The model under review builds one solid part; all positions refer to its coordinate system, in mm. A direction names the side the tool comes from. Give positions to 0.01 mm unless a question says otherwise; leave off trailing zeros. Order: outer loops, then holes, each group sorted by start corner. A loop starts at its lowest first (then second) coordinate and runs counter-clockwise, first axis right, second up. Notation, with made-up numbers: (24.5, -2.75) -> (57.5, -2.75) arc R15 cw to (57.5, 9.25) -> close; hole circle Ø10 at (24, 55). An arc over 180 degrees is marked (long way). Use one line per item in the form item = value.
```python
from build123d import *

# Parameters (mm, degrees)
SKETCH1_W           = 35
SKETCH1_H           = 35
BOSS_EXTRUDE1_DEPTH = 9
SKETCH2_W           = 2
SKETCH2_H           = 35
SKETCH2_W_2         = 1.8
CUT_EXTRUDE1_DEPTH  = 3
SKETCH3_W           = 35
SKETCH3_H           = 3
CUT_EXTRUDE2_DEPTH  = 3
SKETCH4_W           = 7
SKETCH4_H           = 2.65
CUT_EXTRUDE3_DEPTH  = 51.309044912
SKETCH5_W           = 32
SKETCH5_H           = 3
CUT_EXTRUDE4_DEPTH  = 3
SKETCH6_W           = 17.8
SKETCH6_H           = 2
CUT_EXTRUDE5_DEPTH  = 3
SKETCH7_W           = 1.5
SKETCH7_H           = 2.079992284
SKETCH7_H_2         = 2.089639239
SKETCH7_H_3         = 2.130315237
SKETCH7_H_4         = 2.284421
SKETCH7_H_5         = 1.923722947
SKETCH7_H_6         = 2.10231694
SKETCH7_H_7         = 1.921766709
CUT_EXTRUDE6_DEPTH  = 3
SKETCH8_W           = 1.5
SKETCH8_H           = 1.855781426
SKETCH8_H_2         = 1.933933062
SKETCH8_H_3         = 1.973134408
SKETCH8_H_4         = 2.021952678
SKETCH8_H_5         = 2.006089453
SKETCH8_H_6         = 2.101240168
SKETCH8_H_7         = 2.045740356
CUT_EXTRUDE7_DEPTH  = 3
SKETCH9_W           = 32
SKETCH9_H           = 3
CUT_EXTRUDE9_DEPTH  = 3
SKETCH11_W          = 29
SKETCH11_H          = 3
CUT_EXTRUDE10_DEPTH = 3


with BuildPart() as part:
    # Sketch1 → Boss-Extrude1 (new body)
    with BuildSketch(Plane(origin=(0, 0, 0), x_dir=(1, 0, 0), z_dir=(0, 1, 0))):
        with Locations((17.5, 17.5)):
            Rectangle(SKETCH1_W, SKETCH1_H)
    extrude(amount=BOSS_EXTRUDE1_DEPTH)

    # Sketch2 → Cut-Extrude1 (cut)
    with BuildSketch(Plane(origin=(0, 9, 0), x_dir=(1, 0, 0), z_dir=(0, 1, 0))):
        with Locations((34, 17.5)):
            Rectangle(SKETCH2_W, SKETCH2_H)
        with Locations((30.6, 17.5)):
            Rectangle(SKETCH2_W_2, SKETCH2_H)
        with Locations((27.3, 17.5)):
            Rectangle(SKETCH2_W_2, SKETCH2_H)
        with Locations((1, 17.5)):
            Rectangle(SKETCH2_W, SKETCH2_H)
        with Locations((4.4, 17.5)):
            Rectangle(SKETCH2_W_2, SKETCH2_H)
        with Locations((7.7, 17.5)):
            Rectangle(SKETCH2_W_2, SKETCH2_H)
    extrude(amount=-CUT_EXTRUDE1_DEPTH, mode=Mode.SUBTRACT)

    # Sketch3 → Cut-Extrude2 (cut)
    with BuildSketch(Plane(origin=(35, 0, 0), x_dir=(0, 0, -1), z_dir=(1, 0, 0))):
        with Locations((17.5, 2)):
            Rectangle(SKETCH3_W, SKETCH3_H)
    extrude(amount=-CUT_EXTRUDE2_DEPTH, mode=Mode.SUBTRACT)

    # Sketch4 → Cut-Extrude3 (cut, through all)
    with BuildSketch(Plane.XY):
        with Locations((22.9, 7.387674937)):
            Rectangle(SKETCH4_W, SKETCH4_H)
        with Locations((12.1, 7.318212489)):
            Rectangle(SKETCH4_W, SKETCH4_H)
    extrude(amount=-CUT_EXTRUDE3_DEPTH, mode=Mode.SUBTRACT)

    # Sketch5 → Cut-Extrude4 (cut)
    with BuildSketch(Plane.XY):
        with Locations((16, 2)):
            Rectangle(SKETCH5_W, SKETCH5_H)
    extrude(amount=-CUT_EXTRUDE4_DEPTH, mode=Mode.SUBTRACT)

    # Sketch6 → Cut-Extrude5 (cut)
    with BuildSketch(Plane(origin=(0, 9, 0), x_dir=(1, 0, 0), z_dir=(0, 1, 0))):
        with Locations((17.5, 4)):
            Rectangle(SKETCH6_W, SKETCH6_H)
        with Locations((17.5, 9)):
            Rectangle(SKETCH6_W, SKETCH6_H)
        with Locations((17.5, 31)):
            Rectangle(SKETCH6_W, SKETCH6_H)
        with Locations((17.5, 26)):
            Rectangle(SKETCH6_W, SKETCH6_H)
    extrude(amount=-CUT_EXTRUDE5_DEPTH, mode=Mode.SUBTRACT)

    # Sketch7 → Cut-Extrude6 (cut)
    with BuildSketch(Plane(origin=(0, 9, 0), x_dir=(1, 0, 0), z_dir=(0, 1, 0))):
        with Locations((6.05, 25.936938184)):
            Rectangle(SKETCH7_W, SKETCH7_H)
        with Locations((2.75, 25.861771744)):
            Rectangle(SKETCH7_W, SKETCH7_H_2)
        with Locations((6.05, 30.892822657)):
            Rectangle(SKETCH7_W, SKETCH7_H_3)
        with Locations((2.75, 30.815769775)):
            Rectangle(SKETCH7_W, SKETCH7_H_4)
        with Locations((28.95, 30.996118802)):
            Rectangle(SKETCH7_W, SKETCH7_H_5)
        with Locations((32.25, 30.996118802)):
            Rectangle(SKETCH7_W, SKETCH7_H_5)
        with Locations((28.95, 25.828744005)):
            Rectangle(SKETCH7_W, SKETCH7_H_6)
        with Locations((32.25, 25.738468889)):
            Rectangle(SKETCH7_W, SKETCH7_H_7)
    extrude(amount=-CUT_EXTRUDE6_DEPTH, mode=Mode.SUBTRACT)

    # Sketch8 → Cut-Extrude7 (cut)
    with BuildSketch(Plane(origin=(0, 9, 0), x_dir=(1, 0, 0), z_dir=(0, 1, 0))):
        with Locations((28.95, 9.105526505)):
            Rectangle(SKETCH8_W, SKETCH8_H)
        with Locations((32.25, 9.105526505)):
            Rectangle(SKETCH8_W, SKETCH8_H)
        with Locations((32.25, 3.949699522)):
            Rectangle(SKETCH8_W, SKETCH8_H_2)
        with Locations((28.95, 3.95623308)):
            Rectangle(SKETCH8_W, SKETCH8_H_3)
        with Locations((6.05, 3.923953213)):
            Rectangle(SKETCH8_W, SKETCH8_H_4)
        with Locations((6.05, 9.030372491)):
            Rectangle(SKETCH8_W, SKETCH8_H_5)
        with Locations((2.75, 8.982797134)):
            Rectangle(SKETCH8_W, SKETCH8_H_6)
        with Locations((2.75, 3.769333302)):
            Rectangle(SKETCH8_W, SKETCH8_H_7)
    extrude(amount=-CUT_EXTRUDE7_DEPTH, mode=Mode.SUBTRACT)

    # Sketch9 → Cut-Extrude9 (cut)
    with BuildSketch(Plane(origin=(0, 0, -35), x_dir=(-1, 0, 0), z_dir=(0, 0, -1))):
        with Locations((-16, 2)):
            Rectangle(SKETCH9_W, SKETCH9_H)
    extrude(amount=-CUT_EXTRUDE9_DEPTH, mode=Mode.SUBTRACT)

    # Sketch11 → Cut-Extrude10 (cut)
    with BuildSketch(Plane.ZY):
        with Locations((-17.5, 2)):
            Rectangle(SKETCH11_W, SKETCH11_H)
    extrude(amount=-CUT_EXTRUDE10_DEPTH, mode=Mode.SUBTRACT)


solid = part.part
```
1. Add section A-A on x = 8. Give the boundary of the cut face in (y, z), then the cut area to 3 significant figures.
Values:
outline = (0, -35) -> (0.5, -35) -> (0.5, -32) -> (3.5, -32) -> (3.5, -35) -> (6, -35) -> (6, 0) -> (3.5, 0) -> (3.5, -3) -> (0.5, -3) -> (0.5, 0) -> (0, 0) -> close
area = 192 mm^2
2. Add section B-B on x = 15. Count the separate pieces of the cut face and the enclosed holes in it, then the cut area to 3 significant figures.
Values:
separate_pieces = 6
enclosed_holes = 0
area = 201 mm^2
3. Tool access review of faces 4 (the face through (32, 8, -26.699)), 5 (the face through (19.4, 7, -33)), 6 (the face through (3.5, 8, -28)): name each direction out of +Z, -Z, +X, -X, +Y, -Y from which nothing blocks a thin tool from reaching the whole face with its end or side.
Values:
face_4 = +X, -X, +Y
face_5 = +Z, -Z
face_6 = +Z, -Z, +Y
4. For L1, parallel to X at y = 7.75, z = -28; L2, parallel to Z at x = 29, y = 6.5; L3, parallel to Y at x = 2, z = -3.5, list the stretches that pass through material, from the lowest coordinate up.
Values:
L1 = 2 to 3.5, 5.3 to 6.8, 15.6 to 19.4, 28.2 to 29.7, 31.5 to 33
L2 = -35 to -31.96, -30.03 to -26.88, -24.78 to -10.03, -8.18 to -4.94, -2.97 to 0
L3 = 0 to 0.5, 3.5 to 6
5. For pin 1 Ø2 at (y, z) = (7.5, -1.5) entering from +X; pin 2 Ø2.5 at (y, z) = (8, -34) entering from -X, all flat-tipped, find the tip position at first contact; note any pin that passes through.
Values:
pin_1 = 33
pin_2 = 2
6. The part is to be moulded in two halves that separate along X. For faces 1 (the face through (2, 8, -33)), 2 (the face through (17, 0, -18)), 3 (the face through (31.5, 8, -7)), say which applies: +X half, -X half, draft (parallel to the pull), parting line (faces both ways), or undercut.
Values:
face_1 = -X half
face_2 = draft
face_3 = undercut
